Autodesk Inventor part; units mm, degrees
ref_plane "YZ Plane" through (0, 0, 0) normal (1, 0, 0) x (0, 1, 0)
ref_plane "XZ Plane" through (0, 0, 0) normal (0, 1, 0) x (-1, 0, 0)
ref_plane "XY Plane" through (0, 0, 0) normal (0, 0, 1) x (1, 0, 0)
sketch "Skizze1" plane through (0, 0, 0) normal (0, 0, 1) x (1, 0, 0)
  line L0 (0, -21) -> (0, 21)
  line L1 (-35, -15) -> (20, -15)
  line L2 (20, 15) -> (-35, 15)
  line L3 (-35, 15) -> (-35, -15)
  line L4 (20, 15) -> (9.0192, 15)
  line L5 (9.0192, -15) -> (20, -15)
  circle A0 centre (20, 0) radius 15
  line L6 (23.3137, 8) -> (28, 3.3137)
  line L7 (28, 3.3137) -> (28, -3.3137)
  line L8 (28, -3.3137) -> (23.3137, -8)
  line L9 (23.3137, -8) -> (16.6863, -8)
  line L10 (16.6863, -8) -> (12, -3.3137)
  line L11 (12, -3.3137) -> (12, 3.3137)
  line L12 (12, 3.3137) -> (16.6863, 8)
  line L13 (16.6863, 8) -> (23.3137, 8)
  line L14 (-49, 0) -> (49, 0)
  point P0 (0, 0)
  point P1 (20, -15)
  point P2 (20, 15)
  point P3 (-3, 0)
  dimension "d18" = 16
extrude "Extrusion1" add sketch "Skizze1" against normal blind 9.7
extrude "Extrusion2" add sketch "Skizze1" against normal blind 10 contours L14 L11 L10 L9 L8 L7 A0 | A0 L14 L7 L6 L13 L12 L11 | L14 L7 L8 L9 L10 L11 | L11 L12 L13 L6 L7 L14
fillet "Rundung1" radius 5 2 edges at (-35, -15, -4.85) (-35, 15, -4.85)
hole "Bohrung1" at (-3, 0, 0) direction (0, 0, -1) diameter 12 end through all
extrude "Extrusion3" add sketch "Skizze1" along normal blind 10.3 contours L14 L11 L10 L9 L8 L7 A0 | A0 L14 L7 L6 L13 L12 L11 | L14 L7 L8 L9 L10 L11 | L11 L12 L13 L6 L7 L14
extrude "Extrusion4" cut sketch "Skizze1" along normal blind 10.3 contours L14 L7 L8 L9 L10 L11 | L11 L12 L13 L6 L7 L14
extrude "Extrusion5" cut sketch "Skizze1" against normal blind 10 contours L14 L7 L8 L9 L10 L11 | L11 L12 L13 L6 L7 L14
properties material "1.0038 S235JR"
Design review of the part built by this model. Coordinates are the model's own, in mm. A direction names the side the tool comes from. Coordinates: 2 decimals unless noted, no trailing zeros. Write each loop counter-clockwise with the first axis right and the second up, starting at its lowest first coordinate (ties: lowest second). Pieces come first, ordered by that corner, then holes.
1) Machinability: for faces 1 (the flat face through (25.69, -5.624, 0.008)), 2 (the flat face through (-35, 0, -5)), which of the approach directions +Z, -Z, +X, -X, +Y, -Y give a long, thin tool a straight path to every point of the face, cutting with its end or side? Answer none if there is none.
2) Add section B-B (z = -7.5). Write out the cut boundary in (x, y).
3) Insertion check: pin 1 (9.5 mm diameter, centred on x = -3, y = 0, fed in from +Z); pin 2 (9 mm diameter, centred on x = -5, y = 0, fed in from -Z); pin 3 (9 mm diameter, centred on x = -11, y = 7, fed in from +Z); pin 4 (1.5 mm diameter, centred on y = 2, z = 5, fed in from -X). Each pin has a flat end and moves straight along its axis. Give the tip position at first contact, or say it passes through.
4) To check wall thickness, follow L1, parallel to X at y = 0, z = -2; L2, parallel to Y at x = -3, z = -7.25; L3, parallel to X at y = -0.25, z = 8.25. State the ranges of each line that lie inside material, in increasing order.
5) Add section C-C (z = 5.25). Write out the cut boundary in (x, y), plus the area to 3 significant figures.
6) Mouldability with a two-part tool opening along Y and no side actions: class faces 3 (the flat face through (14.376, -5.69, 0.292)), 4 (the flat face through (12, 0, 0)), 5 (the flat face through (-14, 0, -9.7)), 6 (the flat face through (-5, -15, -5)) as +Y half, -Y half, draft (parallel to the pull), parting line (faces both ways), or undercut.
7) Add section A-A (y = 0). Write out the cut boundary in (x, z).
8) Add section D-D (x = 13.5). Write out the cut boundary in (y, z), plus the area to 3 significant figures.
Check result:
1. face 1: +Z, -Z
1. face 2: +Z, -Z, -X, +Y, -Y
2. outline: (-35, -10) arc R5 ccw to (-30, -15) - (20, -15) arc R15 ccw to (20, 15) - (-30, 15) arc R5 ccw to (-35, 10) - close; hole circle Ø12 at (-3, 0); hole (12, -3.31) - (16.69, -8) - (23.31, -8) - (28, -3.31) - (28, 3.31) - (23.31, 8) - (16.69, 8) - (12, 3.31) - close
3. pin 1: passes through
3. pin 2: stops at z = -9.7
3. pin 3: stops at z = 0
3. pin 4: stops at x = 5.05
4. L1: x = -35 to -9, 3 to 12, 28 to 35
4. L2: y = -15 to -6, 6 to 15
4. L3: x = 5 to 12, 28 to 35
5. outline: circle Ø30 at (20, 0); hole (12, -3.31) - (16.69, -8) - (23.31, -8) - (28, -3.31) - (28, 3.31) - (23.31, 8) - (16.69, 8) - (12, 3.31) - close
5. area: 495 mm2
6. face 3: undercut
6. face 4: undercut
6. face 5: draft
6. face 6: -Y half
7. outline: (-35, -9.7) - (-9, -9.7) - (-9, 0) - (-35, 0) - close; (3, -9.7) - (5, -9.7) - (5, -10) - (12, -10) - (12, 10.3) - (5, 10.3) - (5, 0) - (3, 0) - close; (28, -10) - (35, -10) - (35, 10.3) - (28, 10.3) - close
8. outline: (-15, -9.7) - (-13.52, -9.7) - (-13.52, -10) - (-4.81, -10) - (-4.81, 10.3) - (-13.52, 10.3) - (-13.52, 0) - (-15, 0) - close; (4.81, -10) - (13.52, -10) - (13.52, -9.7) - (15, -9.7) - (15, 0) - (13.52, 0) - (13.52, 10.3) - (4.81, 10.3) - close
8. area: 382 mm2
